Input: part model. Units: mm. Frame: model coordinates. Face numbers are marked on the shaded views. A direction names the side the tool comes from. Give positions to 0.01 mm unless a question says otherwise; leave off trailing zeros. Loops run counter-clockwise (first coordinate to the right, second up) from the corner with the lowest first, then second, coordinate; pieces in that order, holes last. Notation, with made-up numbers: (-2, 79) - (17, 79) arc R22 cw to (17, 106) - close; hole circle Ø5 at (25, 78). An arc over 180 degrees is marked (long way). Answer as a JSON object with one key per item and string values. Group by question number.
(1) Access query for the marked faces 1 and 2. Directions: +Z, -Z, +X, -X, +Y, -Y. A direction counts if a zero-diameter tool reaches every point of the face in a straight line with its end or side. Return the directions, or none.
(2) Section query A-A (y = -21). Return loops of the section in (x, z) (3 decimals).
(3) Pin query (flat end, axial travel): P1, Ø12, axis at y = -57, z = 21.5, coming from the +X side; P2, Ø7, axis at y = -92.5, z = -2, coming from the +X side; P3, Ø24.5, axis at y = -9.5, z = -31.5, coming from the +X side. Return the tip coordinate at first contact, or that it passes through.
(4) Section query C-C (x = 42). Count the separate pieces of the cut face and the enclosed holes in it, plus the area to 3 significant figures.
(5) Section query B-B (z = 28.5). Return loops of the section in (x, y).
(6) Mould query, pull axis Z, two halves, no side actions, for the marked faces 3, 4, 5 and 6. Classes: +Z half, -Z half, draft (parallel to the pull), parting line (faces both ways), or undercut.
(7) Material intervals for L1, parallel to Z at x = 22.5, y = -14.5 (3 decimals); L2, parallel to Y at x = 76, z = -13.5; L3, parallel to X at y = -10.5, z = 27.5, sorted ascending.
```python
from build123d import *

# Parameters (mm, degrees)
BOSS_EXTRUDE1_DEPTH     = 38.1
CUT_EXTRUDE1_DEPTH      = 142.777171117
CUT_EXTRUDE1_DEPTH_BACK = 142.777171117
SKETCH2_R               = 6.35
SKETCH3_W               = 6.35
SKETCH3_H               = 31.75
CUT_EXTRUDE2_DEPTH      = 25.4
SKETCH4_W               = 6.35
SKETCH4_H               = 24.683418283
CUT_EXTRUDE3_DEPTH      = 124.131068378
FILLET1_R               = 0.8128
CHAMFER1_SIZE           = 1.524


with BuildPart() as part:
    # Sketch1 → Boss-Extrude1 (new, symmetric)
    with BuildSketch(Plane.XY):
        Polygon((88.9, -101.6), (88.9, -76.2), (69.85, -76.2), (69.85, -50.8), (44.45, -25.4), (25.4, -25.4), (25.4, 0), (0, 0), (0, -63.5), (38.1, -101.6), align=None)
    extrude(amount=BOSS_EXTRUDE1_DEPTH, both=True)

    # Sketch2 → Cut-Extrude1 (cut, two sides: drawn at the far end of the back side and taken through both)
    with BuildSketch(Plane(origin=(9.525, 9.525, 0), x_dir=(0, 0, -1), z_dir=(0.7071067811865485, 0.7071067811865466, 0)).offset(-CUT_EXTRUDE1_DEPTH_BACK)):
        with Locations(Location((19.05, -67.35463315, 0), (0, 0, 90))):
            Circle(SKETCH2_R)
        with Locations(Location((-19.05, -67.35463315, 0), (0, 0, 90))):
            Circle(SKETCH2_R)
    extrude(amount=CUT_EXTRUDE1_DEPTH + CUT_EXTRUDE1_DEPTH_BACK, mode=Mode.SUBTRACT)

    # Sketch3 → Cut-Extrude2 (cut)
    with BuildSketch(Plane(origin=(0, 0, 0), x_dir=(1, 0, 0), z_dir=(0, 1, 0))):
        with Locations((22.225, 0)):
            Rectangle(SKETCH3_W, SKETCH3_H)
    extrude(amount=-CUT_EXTRUDE2_DEPTH, mode=Mode.SUBTRACT)

    # Sketch4 → Cut-Extrude3 (cut, through all)
    with BuildSketch(Plane(origin=(0, -76.2, 0), x_dir=(1, 0, 0), z_dir=(0, 1, 0))):
        with Locations((85.725, -3.533290859)):
            Rectangle(SKETCH4_W, SKETCH4_H)
    extrude(amount=-CUT_EXTRUDE3_DEPTH, mode=Mode.SUBTRACT)

    # Fillet1
    fillet1_edges = [part.edges().sort_by_distance(p)[0] for p in [
        (19.05, -12.7, 15.875),
        (19.05, -12.7, -15.875),
        (82.55, -88.9, 15.875),
        (82.55, -88.9, -8.808418283),
    ]]
    fillet(fillet1_edges, radius=FILLET1_R)

    # Chamfer1
    chamfer1_edges = [part.edges().sort_by_distance(p)[0] for p in [
        (61.642045905, -42.592045905, -19.05),
        (20.367045905, -83.867045905, -19.05),
        (61.642045905, -42.592045905, 19.05),
        (20.367045905, -83.867045905, 19.05),
    ]]
    chamfer(chamfer1_edges, length=CHAMFER1_SIZE)


solid = part.part
```
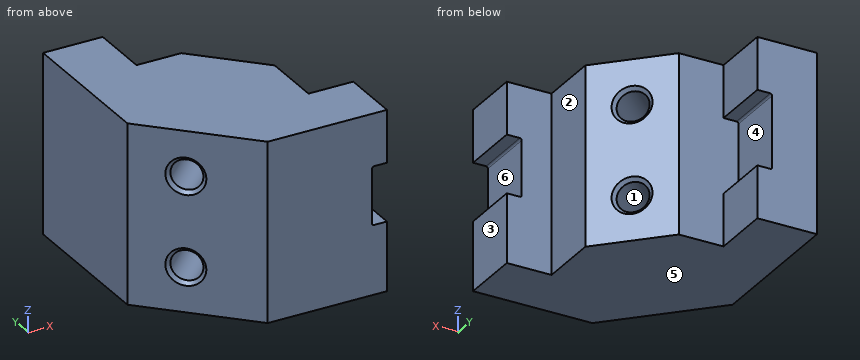
Recorded:
{
 "1": {"face 1": "none", "face 2": "+Z, -Z, +X, +Y"},
 "2": {"outline": "(0, -38.1) - (25.4, -38.1) - (25.4, -15.875) - (19.863, -15.875) arc R0.813 cw to (19.05, -15.062) - (19.05, 15.062) arc R0.813 cw to (19.863, 15.875) - (25.4, 15.875) - (25.4, 38.1) - (0, 38.1) - close"},
 "3": {"P1": "stops at x = 69.85", "P2": "stops at x = 82.55", "P3": "stops at x = 25.4"},
 "4": {"separate pieces": "1", "enclosed holes": "2", "area": "5,450 mm^2"},
 "5": {"outline": "(0, -63.5) - (38.1, -101.6) - (88.9, -101.6) - (88.9, -76.2) - (69.85, -76.2) - (69.85, -50.8) - (44.45, -25.4) - (25.4, -25.4) - (25.4, 0) - (0, 0) - close"},
 "6": {"face 3": "draft", "face 4": "undercut", "face 5": "-Z half", "face 6": "undercut"},
 "7": {"L1": "z = -38.1 to -15.875, 15.875 to 38.1", "L2": "y = -101.6 to -76.2", "L3": "x = 0 to 25.4"}
}
